```python
from build123d import *

# Parameters (mm, degrees)
SKETCH_1_R           = 1.5
EXTRUDE_2_DEPTH      = 50
SKETCH_14_W          = 30
SKETCH_14_H          = 18
CUT_EXTRUDE_6_DEPTH  = 65.195102675
SKETCH_15_W          = 22.4475894
SKETCH_15_H          = 16.25
CUT_EXTRUDE_7_DEPTH  = 30
SKETCH_17_W          = 25.359818697
SKETCH_17_H          = 19
CUT_EXTRUDE_9_DEPTH  = 30
FILLET_8_R           = 10
SKETCH_19_W          = 34.027540403
SKETCH_19_H          = 5
CUT_EXTRUDE_11_DEPTH = 65.759348106
FILLET_9_R           = 10
FILLET_11_R          = 10
FILLET_12_R          = 10
CUT_EXTRUDE_12_DEPTH = 3
CUT_EXTRUDE_START    = -5
SKETCH_21_R          = 3
CUT_EXTRUDE_13_DEPTH = 5


with BuildPart() as part:
    # 草图1 → 凸台-拉伸2 (new body)
    with BuildSketch(Plane.XY):
        with BuildLine():
            Line((15.60515688, 4.016530447), (15.60515688, 4.161375168))
            Line((15.60515688, 4.161375168), (-16.917233431, 4.161375168))
            Line((-16.917233431, 4.161375168), (-36.422020871, -9.496024029))
            ThreePointArc((-36.422020871, -9.496024029), (-37.404323302, -15.066937951), (-31.83340938, -16.049240383))
            Line((-31.83340938, -16.049240383), (-14.39484312, -3.838624832))
            Line((-14.39484312, -3.838624832), (15.60515688, -3.838624832))
            Line((15.60515688, -3.838624832), (15.60515688, -3.693780111))
            ThreePointArc((15.60515688, -3.693780111), (20.671823547, 0.161375168), (15.60515688, 4.016530447))
        make_face()
        with Locations((-34.127715125, -12.772632206)):
            Circle(SKETCH_1_R, mode=Mode.SUBTRACT)
        with Locations((16.671823547, 0.161375168)):
            Circle(SKETCH_1_R, mode=Mode.SUBTRACT)
    extrude(amount=EXTRUDE_2_DEPTH)

    # 草图14 → 切除-拉伸6 (cut, through all)
    with BuildSketch(Plane.XZ.offset(3.838624832)):
        with Locations((5.671823547, 41)):
            Rectangle(SKETCH_14_W, SKETCH_14_H)
        with Locations((5.671823547, 9)):
            Rectangle(SKETCH_14_W, SKETCH_14_H)
    extrude(amount=-CUT_EXTRUDE_6_DEPTH, mode=Mode.SUBTRACT)

    # 草图15 → 切除-拉伸7 (cut)
    with BuildSketch(Plane(origin=(0, 4.161375168, 0), x_dir=(1, 0, 0), z_dir=(0, 1, 0))):
        with Locations((-28.141028131, -16.875)):
            Rectangle(SKETCH_15_W, SKETCH_15_H)
    extrude(amount=-CUT_EXTRUDE_7_DEPTH, mode=Mode.SUBTRACT)

    # 草图17 → 切除-拉伸9 (cut)
    with BuildSketch(Plane(origin=(0, 4.161375168, 0), x_dir=(1, 0, 0), z_dir=(0, 1, 0))):
        with Locations((-29.59714278, -34.5)):
            Rectangle(SKETCH_17_W, SKETCH_17_H)
    extrude(amount=-CUT_EXTRUDE_9_DEPTH, mode=Mode.SUBTRACT)

    # 圆角8
    # the kernel refuses this fillet: 10 mm, written as the material it takes off along each edge
    with BuildSketch(Plane(origin=(-16.917233431, -5.604821542, 8.75), x_dir=(0.8191520442889905, 0.573576436351048, 0), z_dir=(0, 0, 1))) as fillet_8_piece_1:
        with BuildLine():
            CenterArc((13.012933373, 1.149926903), FILLET_8_R, 145, 41.603203435)
            Line((4.82141293, 6.885691266), (0, 0))
            Line((0, 0), (3.079269995, 0))
        make_face()
    extrude(amount=35.25, mode=Mode.SUBTRACT)

    # 草图19 → 切除-拉伸11 (cut, through all)
    with BuildSketch(Plane(origin=(-7.520806183, 10.740824359, 0), x_dir=(0.8191520442889908, 0.5735764363510477, 0), z_dir=(-0.5735764363510477, 0.8191520442889908, 0))):
        with Locations((-22.268098274, -2.5)):
            Rectangle(SKETCH_19_W, SKETCH_19_H)
    extrude(amount=-CUT_EXTRUDE_11_DEPTH, mode=Mode.SUBTRACT)

    # 圆角9
    fillet_9_edges = [part.edges().sort_by_distance(p)[0] for p in [
        (-9.328176453, 0.161375168, 18),
        (-9.328176453, 0.161375168, 32),
    ]]
    fillet(fillet_9_edges, radius=FILLET_9_R)

    # 圆角11
    # the kernel refuses this fillet: 10 mm, written as the material it adds along each edge
    with BuildSketch(Plane(origin=(-16.917233431, 29.161375168, 44), x_dir=(0, 0, -1), z_dir=(0, -1, 0))) as fillet_11_piece_1_section:
        with BuildLine():
            CenterArc((FILLET_11_R, -FILLET_11_R), FILLET_11_R, 90, 90)
            Line((0, -FILLET_11_R), (0, 0))
            Line((0, 0), (FILLET_11_R, 0))
        make_face()
    fillet_11_piece_1 = extrude(amount=26.360319786, mode=Mode.PRIVATE)
    fillet_11_piece_1 = split(fillet_11_piece_1, bisect_by=Plane(origin=(-17.705446038, 3.609462759, 40.498761656), z_dir=(0.5735764363510475, -0.8191520442889908, 0)), keep=Keep.TOP, mode=Mode.PRIVATE)
    add(fillet_11_piece_1)
    with BuildSketch(Plane(origin=(-16.917233431, 29.161375168, 8.75), x_dir=(-1, 0, 0), z_dir=(0, -1, 0))) as fillet_11_piece_2_section:
        with BuildLine():
            CenterArc((FILLET_11_R, -FILLET_11_R), FILLET_11_R, 90, 90)
            Line((0, -FILLET_11_R), (0, 0))
            Line((0, 0), (FILLET_11_R, 0))
        make_face()
    fillet_11_piece_2 = extrude(amount=26.360319786, mode=Mode.PRIVATE)
    fillet_11_piece_2 = split(fillet_11_piece_2, bisect_by=Plane(origin=(-17.705446038, 3.609462759, 12.251238344), z_dir=(0.5735764363510475, -0.8191520442889908, 0)), keep=Keep.TOP, mode=Mode.PRIVATE)
    add(fillet_11_piece_2)
    with BuildSketch(Plane(origin=(-6.917233431, 2.801055382, 8.75), x_dir=(-1, 0, 0), z_dir=(0, 1, 0))) as fillet_11_piece_3_section:
        with BuildLine():
            CenterArc((10 + FILLET_11_R, FILLET_11_R), FILLET_11_R, 180, 90)
            Line((10 + FILLET_11_R, 0), (10, 0))
            Line((10, 0), (10, FILLET_11_R))
        make_face()
    fillet_11_piece_3 = revolve(axis=Axis((-6.917233431, 2.801055382, 8.75), (0, 0, 1)), revolution_arc=184.854944875, mode=Mode.PRIVATE)
    fillet_11_piece_3 = split(fillet_11_piece_3, bisect_by=Plane(origin=(-14.201650521, -3.703349918, 18.374598869), z_dir=(-0.5735764363510472, 0.819152044288991, 0)), keep=Keep.TOP, mode=Mode.PRIVATE)
    fillet_11_piece_3 = split(fillet_11_piece_3, bisect_by=Plane(origin=(-18.790262012, 2.849866436, 18.374598869), z_dir=(0.5735764363510475, -0.8191520442889908, 0)), keep=Keep.TOP, mode=Mode.PRIVATE)
    add(fillet_11_piece_3)
    with BuildSketch(Plane(origin=(-6.917233431, 2.801055382, 44), x_dir=(-1, 0, 0), z_dir=(0, 1, 0))) as fillet_11_piece_4_section:
        with BuildLine():
            CenterArc((10 + FILLET_11_R, -FILLET_11_R), FILLET_11_R, 90, 90)
            Line((10 + FILLET_11_R, 0), (10, 0))
            Line((10, 0), (10, -FILLET_11_R))
        make_face()
    fillet_11_piece_4 = revolve(axis=Axis((-6.917233431, 2.801055382, 44), (0, 0, 1)), revolution_arc=184.854944875, mode=Mode.PRIVATE)
    fillet_11_piece_4 = split(fillet_11_piece_4, bisect_by=Plane(origin=(-14.743190126, -4.082540032, 40.444195091), z_dir=(-0.5735764363510472, 0.819152044288991, 0)), keep=Keep.TOP, mode=Mode.PRIVATE)
    fillet_11_piece_4 = split(fillet_11_piece_4, bisect_by=Plane(origin=(-19.331801617, 2.470676322, 40.444195091), z_dir=(0.5735764363510475, -0.8191520442889908, 0)), keep=Keep.TOP, mode=Mode.PRIVATE)
    add(fillet_11_piece_4)

    # 圆角12
    # the kernel refuses this fillet: 10 mm, written as the material it takes off along each edge
    with BuildSketch(Plane(origin=(-9.328176453, -28.587996687, 50), x_dir=(-1, 0, 0), z_dir=(0, 1, 0))) as fillet_12_piece_1:
        with BuildLine():
            CenterArc((9.899748742, -10), FILLET_12_R, 90, 84.260829523)
            Line((-0.050125629, -9), (-1.045113066, -8.9))
            ThreePointArc((-1.045113066, -8.9), (-1, -8), (-1, 0))
            Line((-1, 0), (0, 1))
            Line((0, 1), (9.899748742, 1))
            Line((9.899748742, 1), (9.899748742, 0))
        make_face()
    extrude(amount=57.498743711, mode=Mode.SUBTRACT)
    with BuildSketch(Plane(origin=(-9.328176453, -25.67610982, 5), x_dir=(-1, 0, 0), z_dir=(0, 1, 0))) as fillet_12_piece_2:
        with BuildLine():
            CenterArc((8.734993995, 10), FILLET_12_R, 200.487315115, 69.512684885)
            Line((-0.632503002, 6.5), (-1.569252702, 6.15))
            ThreePointArc((-1.569252702, 6.15), (-1, 3), (-1, 0))
            Line((-1, 0), (0, -1))
            Line((0, -1), (8.734993995, -1))
            Line((8.734993995, -1), (8.734993995, 0))
        make_face()
    extrude(amount=51.674969976, mode=Mode.SUBTRACT)

    # 草图20 → 切除-拉伸12 (cut)
    with BuildSketch(Plane.XY.offset(50)):
        with BuildLine():
            Line((-35.848444434, -10.315176073), (-19.465403549, 1.156352654))
            ThreePointArc((-19.465403549, 1.156352654), (-15.287218107, 0.41962583), (-16.02394493, -3.758559612))
            Line((-16.02394493, -3.758559612), (-32.406985816, -15.230088339))
            ThreePointArc((-32.406985816, -15.230088339), (-36.585171258, -14.493361515), (-35.848444434, -10.315176073))
        make_face()
    extrude(amount=-CUT_EXTRUDE_12_DEPTH, mode=Mode.SUBTRACT)

    # 草图21 → 切除-拉伸13 (cut)
    with BuildSketch(Plane(origin=(0, 0, 44), x_dir=(-1, 0, 0), z_dir=(0, 0, -1)).offset(CUT_EXTRUDE_START)):
        with Locations(Location((34.127715125, -12.772632206, 0), (0, 0, 235))):
            Circle(SKETCH_21_R)
    extrude(amount=CUT_EXTRUDE_13_DEPTH, mode=Mode.SUBTRACT)


with BuildPart() as body_2:
    # 镜向1: mirrored copy
    add(part.part.mirror(Plane.ZX.offset(14.161375168)))


solid = body_2.part
```
Build history of the part. All positions in model axes, mm. A direction names the side the tool comes from. Give positions to 0.01 mm unless a question says otherwise; leave off trailing zeros. Order: outer loops, then holes, each group sorted by start corner. A loop starts at its lowest first (then second) coordinate and runs counter-clockwise, first axis right, second up. Notation, with made-up numbers: M 64,81.25 L 85,81.25 A11 cw 85,86.25 Z; hole C -26,69.25 d10. An arc over 180 degrees is marked long. Write item = value, one per line. Start each with the question number.
(1) Slice it at A-A on z = 28. Write the cut outline in (x, y), plus the area to 3 significant figures.
(2) Slice it at D-D on z = 45. Write the cut outline in (x, y), plus the area to 3 significant figures.
(3) Which spindle directions (+Z, -Z, +X, -X, +Y, -Y) get a long thin tool onto all of the face, cutting with end or side? Do faces 4 (the cylindrical face through (-17.23, 24.98, 16.27)), 5 (the flat face through (11, 28, 18)), 6 (the flat face through (-27.8, 33, 48.5)). Say none if no direction does.
(4) Two-plate mould, pull along Z, no slides. Class faces 1 (the flat face through (11, 28, 32)), 2 (the flat face through (-16.917, 25, 26)), 3 (the flat face through (-3, 32.161, 27)): released by +Z, released by -Z, zero draft, split by the parting line, or undercut.
(5) Probe L1, parallel to Y at x = 2, z = 25; L2, parallel to Z at x = -25.5, y = 37.5; L3, parallel to Z at x = 13, y = 25.75. List the from-to ranges inside material, lowest first. Write a range as [from, to].
(6) Slice it at B-B on z = 39. Write the cut outline in (x, y).
(7) Slice it at C-C on x = -8. Write the cut outline in (y, z).
(8) Pin check, flat tips, straight feed: pin 1 Ø4 at (x, z) = (-14, 43) entering from +Y; pin 2 Ø2 at (x, y) = (-10.5, 34.5) entering from -Z; pin 3 Ø1.1 at (y, z) = (25, 26.5) entering from -X; pin 4 Ø3 at (x, z) = (-11, 41) entering from +Y. Stop position of each tip, or through.
Responses:
q1.outline = M -16.92,24.16 L 15.61,24.16 L 15.61,24.31 A4 ccw long 15.61,32.02 L 15.61,32.16 L -14.39,32.16 A10 ccw -16.92,25.52 Z; hole C 16.67,28.16 d3
q1.area = 281 mm2
q2.outline = M -36.42,37.82 L -16.92,24.16 L -10.57,24.16 L -10.57,32.16 L -14.39,32.16 L -31.83,44.37 A4 ccw Z; hole C -34.13,41.1 d6
q2.area = 218 mm2
q3.face_4 = -X, +Y, -Y
q3.face_5 = -Z, +X, +Y, -Y
q3.face_6 = +Z
q4.face_1 = released by +Z
q4.face_2 = undercut
q4.face_3 = zero draft
q5.L1 = [24.16, 32.16]
q5.L2 = [5, 8.75], [44, 47]
q5.L3 = [18, 32]
q6.outline = M -18.26,25.1 L -16.92,24.16 L -8.87,24.16 L -8.87,32.16 L -14.39,32.16 L -15.5,32.93 A11.34 ccw -18.26,25.52 Z
q7.outline = M 24.16,12.98 L 32.16,12.98 L 32.16,37.02 L 24.16,37.02 Z
q8.pin_1 = 33.29
q8.pin_2 = through
q8.pin_3 = -16.92
q8.pin_4 = 32.16
